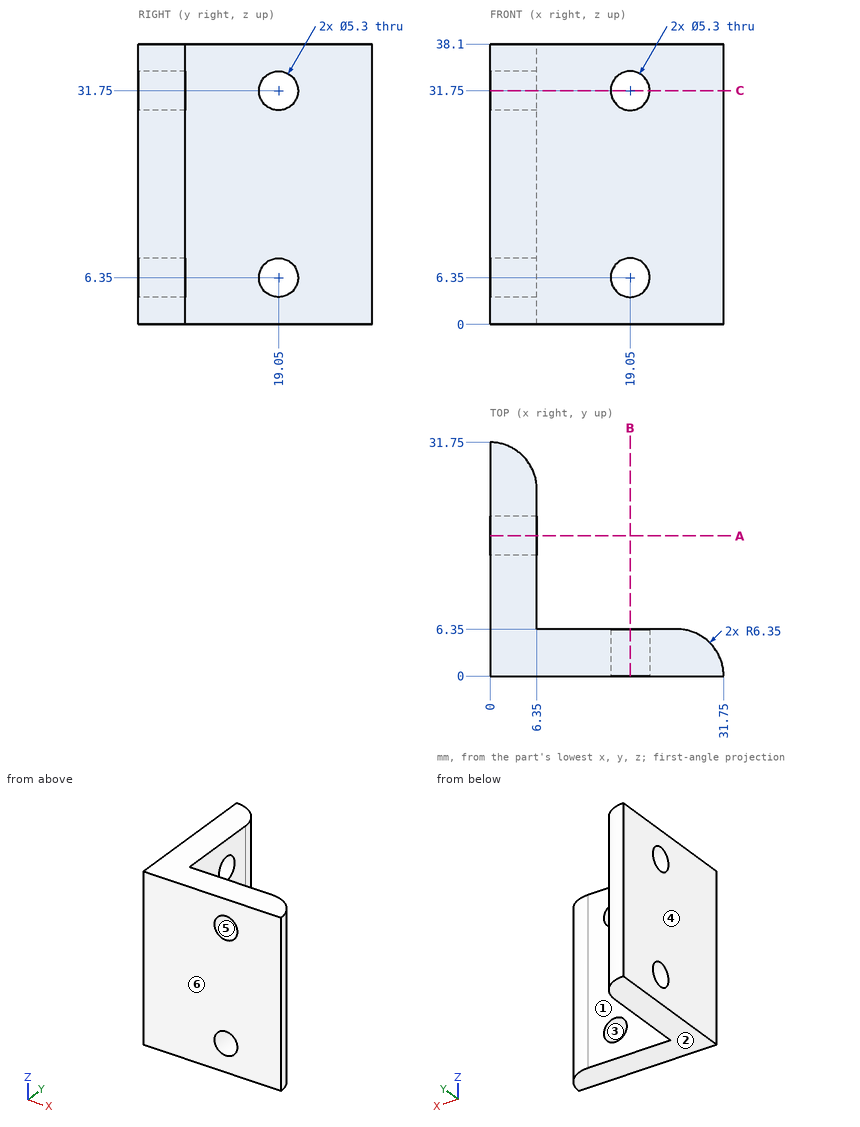
Geometry check sheet. Reference: drawing and pictorial views, mm from the part's lowest x, y, z. A direction names the side the tool comes from. Coordinates: 2 decimals unless noted, no trailing zeros. Write each loop counter-clockwise with the first axis right and the second up, starting at its lowest first coordinate (ties: lowest second). Pieces come first, ordered by that corner, then holes. Notation, with made-up numbers: M 85.25,65 L 107.25,65 A23 cw 107.25,96 Z; hole C 50.5,65.5 d1. An arc over 180 degrees is marked long. Use one line per item in the form item = value.
Item 1: Sectioned sample at C-C, the plane z = 31.75. State how many separate pieces and enclosed holes the cut face has, and give its area (3 significant figures).
Answer below:
separate_pieces = 3
enclosed_holes = 0
area = 278 mm^2
Item 2: Release check for a two-part mould opening along X. For the marked faces 3, 4, 5 and 6 record: pulls with the +X half, pulls with the -X half, needs draft (parallel to the pull), parting line crosses it, or undercut.
Answer below:
face_3 = undercut
face_4 = pulls with the -X half
face_5 = undercut
face_6 = needs draft
Item 3: Material ranges on L1, parallel to Z at x = 19, y = 2; L2, parallel to Y at x = 7, z = 22, recorded low to high. Write a range as from..to.
Answer below:
L1 = 0..3.7, 9..29.1, 34.4..38.1
L2 = 0..6.35
Item 4: Gauge pin test, flat ends, axial feed: pin 1 Ø4 at (x, z) = (19.05, 31.75) entering from +Y; pin 2 Ø15 at (y, z) = (20.5, 24.5) entering from +X; pin 3 Ø5.5 at (x, z) = (15, 16) entering from +Y. Record the tip position at first contact, or that the pin passes through.
Answer below:
pin_1 = through
pin_2 = 6.35
pin_3 = 6.35
Item 5: Set-up check for the marked faces 1 and 2: record each of +Z, -Z, +X, -X, +Y, -Y from which the full face is reachable in a straight line by a thin tool's end or side.
Answer below:
face_1 = +Z, -Z, +X, +Y
face_2 = -Z, +X, -X, +Y, -Y
Item 6: Sectioned sample at A-A, the plane y = 19.05. Record the cut outline in (x, z), and give its area (3 significant figures).
Answer below:
outline = M 0,0 L 6.35,0 L 6.35,3.7 L 0,3.7 Z; M 0,9 L 6.35,9 L 6.35,29.1 L 0,29.1 Z; M 0,34.4 L 6.35,34.4 L 6.35,38.1 L 0,38.1 Z
area = 175 mm^2
